The figure shows three views and two pictorial views of one solid part (mm, origin at its lowest corner). Answer the questions. Coordinates: 2 decimals unless noted, no trailing zeros. Write each loop counter-clockwise with the first axis right and the second up, starting at its lowest first coordinate (ties: lowest second). Pieces come first, ordered by that corner, then holes.
Item 1: Section C-C (y = 4.25) is taken. Give the vertices of the cut face in (x, z), then the cut area to 3 significant figures.
Item 2: Each of these flat-tipped pins is pushed along its axis until it touches: P1, Ø5, axis at x = 38.1, z = 38.1, coming from the +Y side; P2, Ø10, axis at x = 48.5, y = 20, coming from the -Z side; P3, Ø8, axis at y = 3.5, z = 17, coming from the +X side; P4, Ø12, axis at x = 9, z = 22.5, coming from the -Y side. Where does it stop, or does it pass through?
Item 3: Section D-D (y = 15) is taken. Give the vertices of the cut face in (x, z).
Item 4: Determine the mould class of the marked faces 1, 2 and 3 for opening direction X: released by +X, released by -X, zero draft, split by the parting line, or undercut.
Item 5: Straight lines are drawn through the part: probe 1 along X at (y, z) = (4.5, 38.1); probe 2 along X at (y, z) = (20.25, 39) (1 decimal); probe 3 along Y at (x, z) = (15, 60.5). For each, find the intervals that lie inside material, in ascending order.
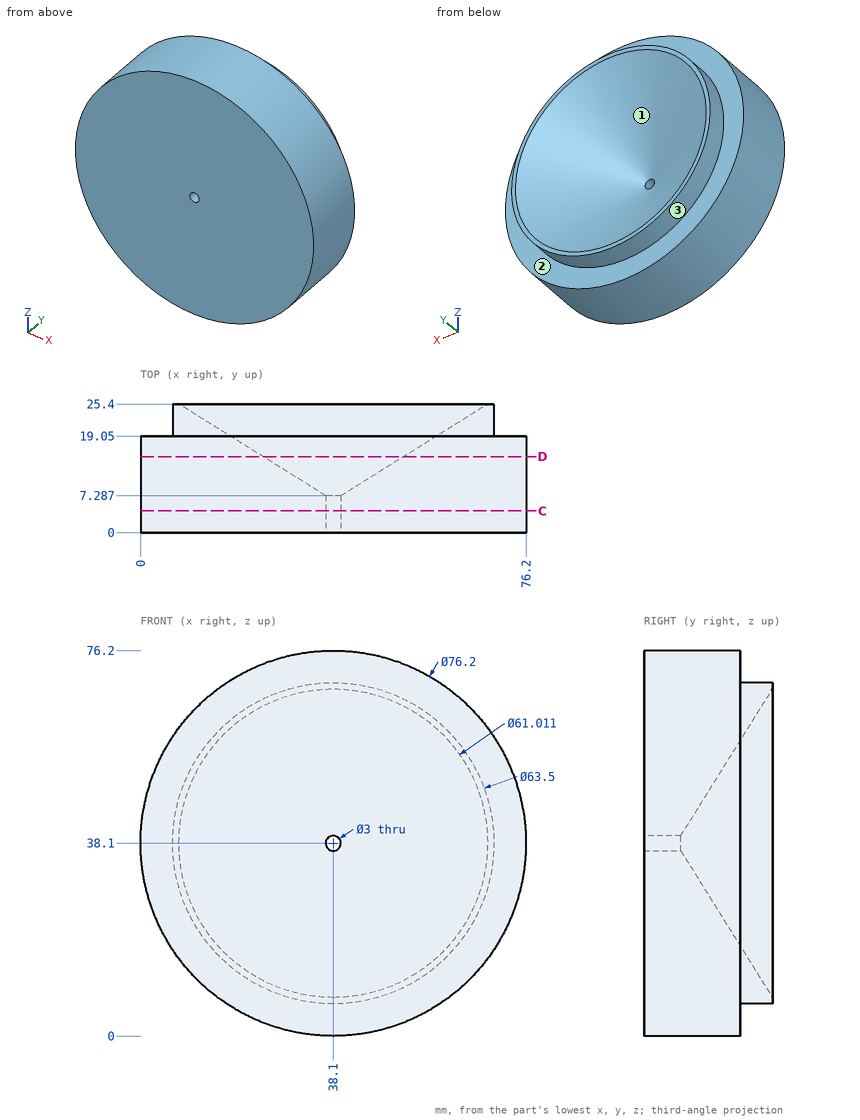
Established:
1. outline: circle Ø76.2 at (38.1, 38.1); hole circle Ø3 at (38.1, 38.1)
1. area: 4,550 mm2
2. P1: stops at y = 7.91
2. P2: stops at z = 0.4
2. P3: stops at x = 72.15
2. P4: stops at y = 0
3. outline: circle Ø76.2 at (38.1, 38.1); hole circle Ø27.7 at (38.1, 38.1)
4. face 1: undercut
4. face 2: zero draft
4. face 3: split by the parting line
5. probe 1: x = 0 to 36.6, 39.6 to 76.2
5. probe 2: x = 6.4 to 15.9, 60.3 to 69.8
5. probe 3: y = 0 to 19.05
